```python
from build123d import *

# Parameters (mm, degrees)
SKETCH_1_W          = 94
SKETCH_1_H          = 64
EXTRUDE_1_DEPTH     = 7
FILLET_1_R          = 1
SKETCH_2_W          = 86
SKETCH_2_H          = 57
CUT_EXTRUDE_1_DEPTH = 5
SKETCH_3_R          = 1.55
CUT_EXTRUDE_2_DEPTH = 58.28874235
SKETCH_4_W          = 20
SKETCH_4_H          = 5
CUT_EXTRUDE_4_DEPTH = 5


with BuildPart() as part:
    # 草图1 → 凸台-拉伸1 (new body)
    with BuildSketch(Plane.XY):
        Rectangle(SKETCH_1_W, SKETCH_1_H)
    extrude(amount=EXTRUDE_1_DEPTH)

    # 圆角1
    fillet_1_edges = [part.edges().sort_by_distance(p)[0] for p in [
        (47, -32, 3.5),
        (-47, -32, 3.5),
        (-47, 32, 3.5),
        (47, 32, 3.5),
    ]]
    fillet(fillet_1_edges, radius=FILLET_1_R)

    # 草图2 → 切除-拉伸1 (cut)
    with BuildSketch(Plane.XY.offset(7)):
        Rectangle(SKETCH_2_W, SKETCH_2_H)
    extrude(amount=-CUT_EXTRUDE_1_DEPTH, mode=Mode.SUBTRACT)

    # 草图3 → 切除-拉伸2 (cut, through all)
    with BuildSketch(Plane.XY.offset(7)):
        with Locations((-44.7, 29.7)):
            Circle(SKETCH_3_R)
        with Locations(Location((44.7, 29.7, 0), (0, 0, 180))):
            Circle(SKETCH_3_R)
        with Locations((44.7, -29.7)):
            Circle(SKETCH_3_R)
        with Locations(Location((-44.7, -29.7, 0), (0, 0, 180))):
            Circle(SKETCH_3_R)
    extrude(amount=-CUT_EXTRUDE_2_DEPTH, mode=Mode.SUBTRACT)

    # 草图4 → 切除-拉伸4 (cut)
    with BuildSketch(Plane.XZ.offset(32)):
        with Locations((7.68, 5.5)):
            Rectangle(SKETCH_4_W, SKETCH_4_H)
    extrude(amount=-CUT_EXTRUDE_4_DEPTH, mode=Mode.SUBTRACT)


solid = part.part
```
Design review of the part built by this model. Coordinates are the model's own, in mm. A direction names the side the tool comes from. Coordinates: 2 decimals unless noted, no trailing zeros. Order: outer loops, then holes, each group sorted by start corner. A loop starts at its lowest first (then second) coordinate and runs counter-clockwise, first axis right, second up. Notation, with made-up numbers: M 34,82 L 56,82 A20 cw 56,94 Z; hole C -15.5,-19.5 d8. An arc over 180 degrees is marked long. Answer as a JSON object with one key per item and string values. Group by question number.
1) Add section D-D, the plane y = -29.7. Write out the cut boundary in (x, z).
2) Tool access review of faces 1 (the flat face through (-1, 32, 3)), 2 (the flat face through (8, -30, 3)), 3 (the flat face through (-1, 0, 2)): name each direction out of +Z, -Z, +X, -X, +Y, -Y from which nothing blocks a thin tool from reaching the whole face with its end or side.
3) For pin 1 (2 mm diameter, centred on x = -34, y = 19.5, fed in from +Z); pin 2 (1.9 mm diameter, centred on x = 44.7, y = -29.7, fed in from -Z); pin 3 (1 mm diameter, centred on x = 10, y = -31, fed in from +Z), all flat-tipped, find the tip position at first contact; note any pin that passes through.
4) Add section B-B, the plane y = 29.7. Write out the cut boundary in (x, z).
5) Add section A-A, the plane x = -44.7. Write out the cut boundary in (y, z), then the cut area to 3 significant figures.
6) Add section C-C, the plane z = 4.75. Write out the cut boundary in (x, y).
7) Wall thickness on L1, parallel to Y at x = 44.7, z = 3; L2, parallel to X at y = -2, z = 3; L3, parallel to Y at x = -9.5, z = 6: over which ranges is each line inside the solid? List them lowest first.
8) Mouldability with a two-part tool opening along Y and no side actions: class faces 4 (the flat face through (-47, 0, 3)), 5 (the flat face through (-43, 0, 5)), 6 (the flat face through (-0.6, -32, 2.7)) as pulls with the +Y half, pulls with the -Y half, needs draft (parallel to the pull), parting line crosses it, or undercut.
Computed values:
{
 "1": {"outline": "M -47,0 L -46.25,0 L -46.25,7 L -47,7 Z; M -43.15,0 L 43.15,0 L 43.15,7 L 17.68,7 L 17.68,3 L -2.32,3 L -2.32,7 L -43.15,7 Z; M 46.25,0 L 47,0 L 47,7 L 46.25,7 Z"},
 "2": {"face 1": "+Z, -Z, +X, -X, +Y", "face 2": "+Z, -Y", "face 3": "+Z"},
 "3": {"pin 1": "stops at z = 2", "pin 2": "passes through", "pin 3": "stops at z = 3"},
 "4": {"outline": "M -47,0 L -46.25,0 L -46.25,7 L -47,7 Z; M -43.15,0 L 43.15,0 L 43.15,7 L -43.15,7 Z; M 46.25,0 L 47,0 L 47,7 L 46.25,7 Z"},
 "5": {"outline": "M -32,0 L -31.25,0 L -31.25,7 L -32,7 Z; M -28.15,0 L 28.15,0 L 28.15,7 L -28.15,7 Z; M 31.25,0 L 32,0 L 32,7 L 31.25,7 Z", "area": "405 mm^2"},
 "6": {"outline": "M -47,-31 A1 ccw -46,-32 L -2.32,-32 L -2.32,-28.5 L -43,-28.5 L -43,28.5 L 43,28.5 L 43,-28.5 L 17.68,-28.5 L 17.68,-32 L 46,-32 A1 ccw 47,-31 L 47,31 A1 ccw 46,32 L -46,32 A1 ccw -47,31 Z; hole C -44.7,-29.7 d3.1; hole C -44.7,29.7 d3.1; hole C 44.7,-29.7 d3.1; hole C 44.7,29.7 d3.1"},
 "7": {"L1": "y = -32 to -31.25, -28.15 to 28.15, 31.25 to 32", "L2": "x = -47 to -43, 43 to 47", "L3": "y = -32 to -28.5, 28.5 to 32"},
 "8": {"face 4": "needs draft", "face 5": "undercut", "face 6": "pulls with the -Y half"}
}
